from build123d import *

# Parameters (mm, degrees)
F1_DEPTH  = 4
F2_W      = 15
F2_H      = 5
F2_W_2    = 7
F2_H_2    = 9.45
F3_DEPTH  = 15
F4_SIZE   = 7
F6_DEPTH  = 25
F8_DEPTH  = 25
F10_DEPTH = 50


with BuildPart() as f1:
    # F0 (on Top) → F1 (new body)
    with BuildSketch(Plane.XY):
        with BuildLine():
            Line((20, -22), (20, 22))
            Line((20, 22), (-12, 22))
            ThreePointArc((-12, 22), (-17.6568542495, 19.6568542495), (-20, 14))
            Line((-20, 14), (-1.4962593516, 14.9251870324))
            ThreePointArc((-1.4962593516, 14.9251870324), (-0.7490642542, 14.9812850832), (0, 15))
            ThreePointArc((0, 15), (10.6066017178, 10.6066017178), (15, 0))
            ThreePointArc((15, 0), (10.6066017178, -10.6066017178), (0, -15))
            ThreePointArc((0, -15), (-0.7490642542, -14.9812850832), (-1.4962593516, -14.9251870324))
            Line((-1.4962593516, -14.9251870324), (-20, -14))
            ThreePointArc((-20, -14), (-17.6568542495, -19.6568542495), (-12, -22))
            Line((-12, -22), (20, -22))
        make_face()
        with BuildLine():
            ThreePointArc((2, -17.5), (-1.4142135624, -18.9142135624), (0, -15.5))
            ThreePointArc((0, -15.5), (1.4142135624, -16.0857864376), (2, -17.5))
        make_face(mode=Mode.SUBTRACT)
        with BuildLine():
            ThreePointArc((2, 17.5), (1.4142135624, 16.0857864376), (0, 15.5))
            ThreePointArc((0, 15.5), (-1.4142135624, 18.9142135624), (2, 17.5))
        make_face(mode=Mode.SUBTRACT)
    extrude(amount=F1_DEPTH)

    # F2 (on Top) → F3 (join)
    with BuildSketch(Plane.XY):
        with Locations((27.5, 10.05)):
            Rectangle(F2_W, F2_H)
        with Locations((27.5, -10.05)):
            Rectangle(F2_W, F2_H)
        Polygon((20, 22), (20, 12.55), (35, 12.55), align=None)
        with Locations((16.5, 17.275)):
            Rectangle(F2_W_2, F2_H_2)
        Polygon((35, -12.55), (20, -12.55), (20, -22), align=None)
        with Locations((16.5, -17.275)):
            Rectangle(F2_W_2, F2_H_2)
    extrude(amount=F3_DEPTH)

    # F4
    f4_edges = [f1.edges().sort_by_distance(p)[0] for p in [
        (13, 17.275, 15),
        (13, -17.275, 15),
    ]]
    chamfer(f4_edges, length=F4_SIZE)

    # F5 (on face) → F6 (cut)
    with BuildSketch(Plane.XY.offset(15)):
        Polygon((27.5, 12.55), (35, 12.55), (23.75, 19.6375), (23.75, 12.55), align=None)
    extrude(amount=-F6_DEPTH, mode=Mode.SUBTRACT)

    # F7 (on face) → F8 (cut)
    with BuildSketch(Plane.XY.offset(15)):
        Polygon((23.75, -19.6375), (35, -12.55), (27.5, -12.55), (23.75, -12.55), align=None)
    extrude(amount=-F8_DEPTH, mode=Mode.SUBTRACT)

    # F9 (on face) → F10 (cut)
    with BuildSketch(Plane.XZ.offset(12.55)):
        with BuildLine():
            Line((31.125, 7.5), (29.375, 7.5))
            Line((29.375, 7.5), (29.375, 5.75))
            ThreePointArc((29.375, 5.75), (30.6124368671, 6.2625631329), (31.125, 7.5))
        make_face()
        with BuildLine():
            ThreePointArc((31.125, 7.5), (30.6124368671, 8.7374368671), (29.375, 9.25))
            Line((29.375, 9.25), (29.375, 7.5))
            Line((29.375, 7.5), (31.125, 7.5))
        make_face()
        with BuildLine():
            Line((29.375, 7.5), (29.375, 9.25))
            ThreePointArc((29.375, 9.25), (28.1375631329, 8.7374368671), (27.625, 7.5))
            Line((27.625, 7.5), (29.375, 7.5))
        make_face()
        with BuildLine():
            Line((29.375, 5.75), (29.375, 7.5))
            Line((29.375, 7.5), (27.625, 7.5))
            ThreePointArc((27.625, 7.5), (28.1375631329, 6.2625631329), (29.375, 5.75))
        make_face()
    extrude(amount=-F10_DEPTH, mode=Mode.SUBTRACT)


solid = f1.part
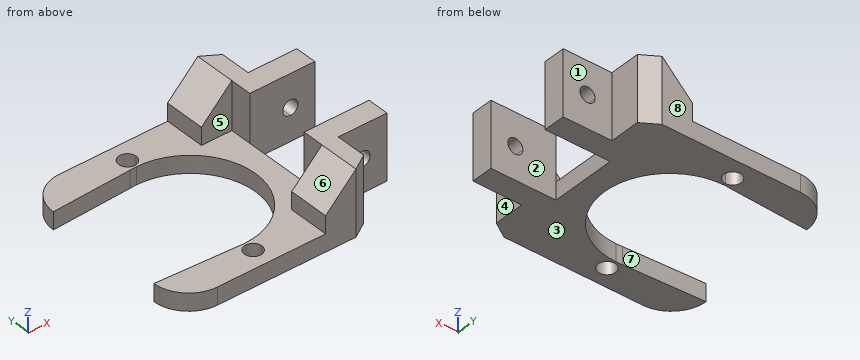
Source: CAD feature listing. Evaluate the final solid. Frame: model axes, mm. Face numbers are marked on the shaded views. A direction names the side the tool comes from. Round coordinates to 2 decimals unless told otherwise and drop trailing zeros. Write each loop counter-clockwise with the first axis right and the second up, starting at its lowest first coordinate (ties: lowest second). Pieces come first, ordered by that corner, then holes. Notation, with made-up numbers: (2.5, 13) - (24.5, 13) arc R33 cw to (24.5, 50) - close; hole circle Ø11 at (-27, 1). An arc over 180 degrees is marked (long way). Use CSV: the item, a comma, the result in double quotes. Start each with the question number.
(1) Mould query, pull axis Y, two halves, no side actions, for the marked faces 6, 7 and 8. Classes: pulls with the +Y half, pulls with the -Y half, needs draft (parallel to the pull), parting line crosses it, or undercut.
(2) Cut plane A-A, the plane z = 13. Return loops of the section in (x, y), and give its area (3 significant figures).
(3) Material intervals for probe 1 along Y at (x, z) = (-1.5, 3.5) (3 decimals); probe 2 along Y at (x, z) = (25.5, 13.75); probe 3 along Y at (x, z) = (14, 8.75), sorted ascending. Write a range as [from, to].
(4) Cut plane D-D, the plane z = 3. Return loops of the section in (x, y).
(5) Set-up query: the marked faces 1, 2, 3, 4 and 5. Return all of +Z, -Z, +X, -X, +Y, -Y with unobstructed straight access to the full face (end or side cutting, diameter ignored); none if empty.
(6) First-contact query: pin 1 Ø1 at (x, y) = (13, -15.5) entering from +Z; pin 2 Ø5.5 at (x, z) = (29.5, 6) entering from -Y; pin 3 Ø1.2 at (y, z) = (15.5, 6.5) entering from -X; pin 4 Ø6 at (y, z) = (-11.5, 5) entering from -X. Flat tips, straight axial feed; report the tip coordinate or a pass-through.
(7) Cut plane C-C, the plane x = 23. Return loops of the section in (y, z), and give its area (3 significant figures).
(8) Cut plane B-B, the plane y = -9. Return loops of the section in (x, z) (3 decimals).
Geometry says:
1,face 6,"needs draft"
1,face 7,"undercut"
1,face 8,"pulls with the +Y half"
2,outline,"(18, -22) - (20, -22) - (23.75, -19.64) - (23.75, -12.55) - (35, -12.55) - (35, -7.55) - (20, -7.55) - (20, -12.55) - (18, -12.55) - close; (18, 12.55) - (20, 12.55) - (20, 7.55) - (35, 7.55) - (35, 12.55) - (23.75, 12.55) - (23.75, 19.64) - (20, 22) - (18, 22) - close"
2,area,"250 mm²"
3,probe 1,"[-22, -18.823], [-16.177, -14.925], [14.925, 16.177], [18.823, 22]"
3,probe 2,"[-12.55, -7.55], [7.55, 12.55]"
3,probe 3,"[-22, -12.55], [12.55, 22]"
4,outline,"(-20, -14) arc R8 ccw to (-12, -22) - (20, -22) - (23.75, -19.64) - (23.75, -12.55) - (35, -12.55) - (35, -7.55) - (20, -7.55) - (20, 7.55) - (35, 7.55) - (35, 12.55) - (23.75, 12.55) - (23.75, 19.64) - (20, 22) - (-12, 22) arc R8 ccw to (-20, 14) - (-1.5, 14.93) arc R15 cw (long way) to (-1.5, -14.93) - close; hole circle Ø4 at (0, -17.5); hole circle Ø4 at (0, 17.5)"
5,face 1,"+Z, -Z, +X, +Y"
5,face 2,"+Z, -Z, +X"
5,face 3,"-Z, +X, -X, +Y, -Y"
5,face 4,"+Z, -Z, +X, -Y"
5,face 5,"+Z, -X"
6,pin 1,"z = 8.5"
6,pin 2,"y = -12.55"
6,pin 3,"x = 13"
6,pin 4,"x = -20"
7,outline,"(-20.11, 0) - (-7.55, 0) - (-7.55, 15) - (-20.11, 15) - close; (7.55, 0) - (20.11, 0) - (20.11, 15) - (7.55, 15) - close"
7,area,"377 mm²"
8,outline,"(12, 0) - (35, 0) - (35, 15) - (20, 15) - (20, 4) - (12, 4) - close; hole circle Ø3.5 at (29.375, 7.5)"
